```python
from build123d import *

# Parameters (mm, degrees)
SKETCH2_W           = 67.5
SKETCH2_H           = 67.5
SKETCH2_R           = 1.5
BOSS_EXTRUDE3_DEPTH = 2
SKETCH1_W           = 32
SKETCH1_H           = 32
SKETCH1_W_2         = 28
SKETCH1_H_2         = 28
BOSS_EXTRUDE4_DEPTH = 17
SKETCH1_6_W         = 49.5
SKETCH1_6_H         = 49.5
SKETCH1_6_W_2       = 45.5
SKETCH1_6_H_2       = 45.5
BOSS_EXTRUDE5_DEPTH = 10


with BuildPart() as part:
    # Sketch2 → Boss-Extrude3 (new body)
    with BuildSketch(Plane(origin=(0, 0, 0), x_dir=(1, 0, 0), z_dir=(0, 1, 0))):
        with Locations((-7.30721393, -10.093283582)):
            Rectangle(SKETCH2_W, SKETCH2_H)
        with Locations(Location((-37.55721393, 20.156716418, 0), (0, 0, 270))):
            Circle(SKETCH2_R, mode=Mode.SUBTRACT)
        with Locations(Location((22.94278607, 20.156716418, 0), (0, 0, 270))):
            Circle(SKETCH2_R, mode=Mode.SUBTRACT)
        with Locations(Location((22.94278607, -40.343283582, 0), (0, 0, 270))):
            Circle(SKETCH2_R, mode=Mode.SUBTRACT)
        with Locations(Location((-37.55721393, -40.343283582, 0), (0, 0, 270))):
            Circle(SKETCH2_R, mode=Mode.SUBTRACT)
    extrude(amount=BOSS_EXTRUDE3_DEPTH)

    # Sketch1 → Boss-Extrude4 (add)
    with BuildSketch(Plane(origin=(0, 0, 0), x_dir=(1, 0, 0), z_dir=(0, 1, 0))):
        with Locations((-7.30721393, -10.093283582)):
            Rectangle(SKETCH1_W, SKETCH1_H)
        with Locations((-7.30721393, -10.093283582)):
            Rectangle(SKETCH1_W_2, SKETCH1_H_2, mode=Mode.SUBTRACT)
    extrude(amount=BOSS_EXTRUDE4_DEPTH)

    # Sketch1_6 → Boss-Extrude5 (add)
    with BuildSketch(Plane(origin=(0, 0, 0), x_dir=(1, 0, 0), z_dir=(0, 1, 0))):
        with Locations((-7.30721393, -10.093283582)):
            Rectangle(SKETCH1_6_W, SKETCH1_6_H)
        with Locations((-7.30721393, -10.093283582)):
            Rectangle(SKETCH1_6_W_2, SKETCH1_6_H_2, mode=Mode.SUBTRACT)
    extrude(amount=BOSS_EXTRUDE5_DEPTH)


solid = part.part
```
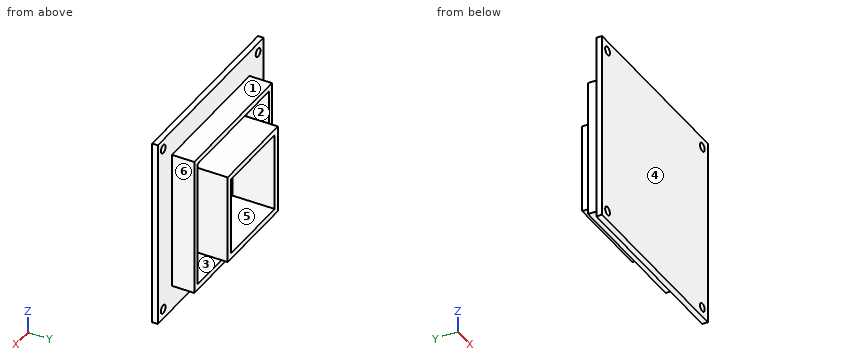
Work out the finished part from the listing and answer in its coordinate system (mm). Face numbers are marked on the shaded views. A direction names the side the tool comes from. Give positions to 0.01 mm unless a question says otherwise; leave off trailing zeros. Order: outer loops, then holes, each group sorted by start corner. A loop starts at its lowest first (then second) coordinate and runs counter-clockwise, first axis right, second up.
1. Section D-D, the plane y = 14.75 is taken. Determine the outline of the cut face in (x, z), and give its area (3 significant figures).
Result sheet:
outline: (-23.31, -5.91) - (8.69, -5.91) - (8.69, 26.09) - (-23.31, 26.09) - close; hole (-21.31, -3.91) - (6.69, -3.91) - (6.69, 24.09) - (-21.31, 24.09) - close
area: 240 mm2
2. The mould has two halves that part along Z. Classify the marked faces 1, 2, 3 and 4: released by +Z, released by -Z, zero draft, split by the parting line, or undercut.
Result sheet:
face 1: released by +Z
face 2: undercut
face 3: undercut
face 4: zero draft
3. Section B-B, the plane z = 1 is taken. Determine the outline of the cut face in (x, y), and give its area (3 significant figures).
Result sheet:
outline: (-41.06, 0) - (26.44, 0) - (26.44, 2) - (17.44, 2) - (17.44, 10) - (15.44, 10) - (15.44, 2) - (8.69, 2) - (8.69, 17) - (6.69, 17) - (6.69, 2) - (-21.31, 2) - (-21.31, 17) - (-23.31, 17) - (-23.31, 2) - (-30.06, 2) - (-30.06, 10) - (-32.06, 10) - (-32.06, 2) - (-41.06, 2) - close
area: 227 mm2
4. Section C-C, the plane x = -16 is taken. Determine the outline of the cut face in (y, z).
Result sheet:
outline: (0, -23.66) - (2, -23.66) - (2, -14.66) - (10, -14.66) - (10, -12.66) - (2, -12.66) - (2, -5.91) - (17, -5.91) - (17, -3.91) - (2, -3.91) - (2, 24.09) - (17, 24.09) - (17, 26.09) - (2, 26.09) - (2, 32.84) - (10, 32.84) - (10, 34.84) - (2, 34.84) - (2, 43.84) - (0, 43.84) - close
5. Section A-A, the plane y = 8.25 is taken. Determine the outline of the cut face in (x, z), and give its area (3 significant figures).
Result sheet:
outline: (-32.06, -14.66) - (17.44, -14.66) - (17.44, 34.84) - (-32.06, 34.84) - close; (-23.31, -5.91) - (8.69, -5.91) - (8.69, 26.09) - (-23.31, 26.09) - close; hole (-30.06, -12.66) - (15.44, -12.66) - (15.44, 32.84) - (-30.06, 32.84) - close; hole (-21.31, -3.91) - (6.69, -3.91) - (6.69, 24.09) - (-21.31, 24.09) - close
area: 620 mm2
6. Straight lines are drawn through the part: L1, parallel to X at y = 9.75, z = 21; L2, parallel to Z at x = -16, y = 8.5; L3, parallel to Z at x = 8.5, y = 6.25. For each, find the intervals that lie inside material, in ascending order.
Result sheet:
L1: x = -32.06 to -30.06, -23.31 to -21.31, 6.69 to 8.69, 15.44 to 17.44
L2: z = -14.66 to -12.66, -5.91 to -3.91, 24.09 to 26.09, 32.84 to 34.84
L3: z = -14.66 to -12.66, -5.91 to 26.09, 32.84 to 34.84
7. Each of these flat-tipped pins is pushed along its axis until it touches: P1, Ø4, axis at x = 2.5, y = 14.5, coming from the -Z side; P2, Ø1, axis at x = -32.5, z = 14, coming from the -Y side; P3, Ø9, axis at y = 7, z = 1, coming from the +X side; P4, Ø1, axis at x = -24, y = 4.5, coming from the +Z side. Where does it stop, or does it pass through?
Result sheet:
P1: stops at z = -5.91
P2: stops at y = 0
P3: stops at x = 17.44
P4: stops at z = 34.84
8. For the marked faces 5 and 6, determine the directions among +Z, -Z, +X, -X, +Y, -Y from which every point of the face is accessible in a straight line to the end or side of a thin tool.
Result sheet:
face 5: +Y
face 6: +Z, -Z, +X, +Y
